Study the drawing (mm; zero at the part's minimum x, y, z) and answer. A direction names the side the tool comes from. Give positions to 0.01 mm unless a question says otherwise; leave off trailing zeros. Write each loop counter-clockwise with the first axis right and the second up, starting at its lowest first coordinate (ties: lowest second). Pieces come first, ordered by that corner, then holes. Notation, with made-up numbers: (-22, 33) - (-13, 33) arc R26 cw to (-13, 62) - close; hole circle Ø11 at (-1.5, -30). An arc over 180 degrees is marked (long way). Return JSON: item names as keys, results as strings.
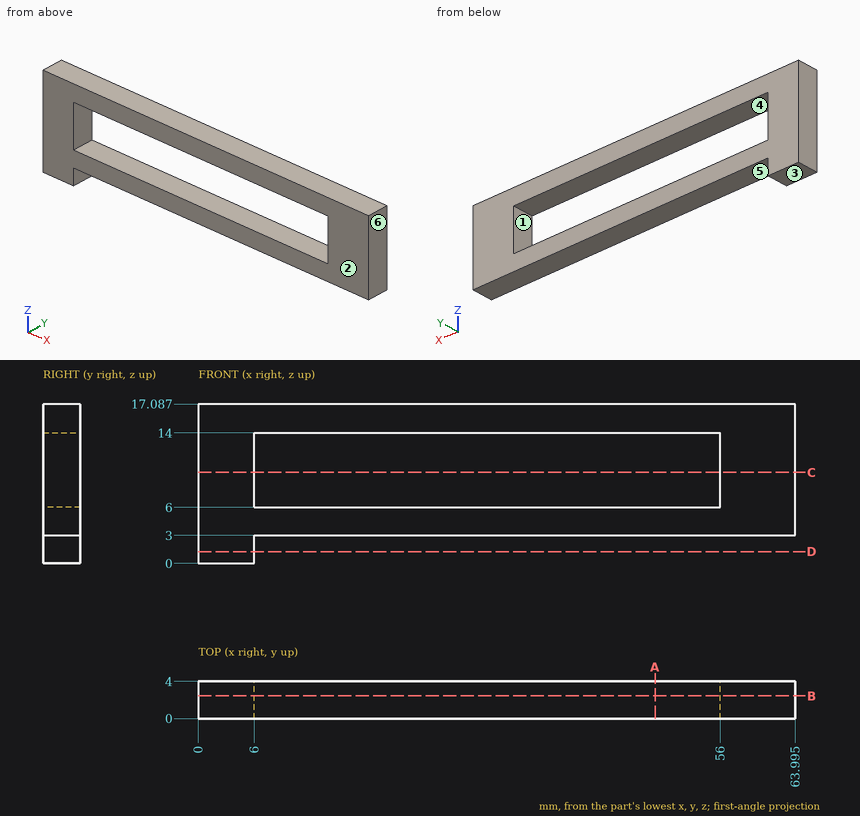
Item 1: The mould has two halves that part along Z. Classify the marked faces 1, 2 and 3: +Z half, -Z half, draft (parallel to the pull), parting line (faces both ways), or undercut.
Answer below:
{"face 1": "undercut", "face 2": "draft", "face 3": "-Z half"}
Item 2: A cutting plane is placed at A-A on x = 49. Determine the outline of the cut face in (y, z).
Answer below:
{"outline": "(0, 3) - (4, 3) - (4, 6) - (0, 6) - close; (0, 14) - (4, 14) - (4, 17.09) - (0, 17.09) - close"}
Item 3: A cutting plane is placed at B-B on y = 2.45. Determine the outline of the cut face in (x, z) (1 decimal).
Answer below:
{"outline": "(0, 0) - (6, 0) - (6, 3) - (64, 3) - (64, 17.1) - (0, 17.1) - close; hole (6, 6) - (56, 6) - (56, 14) - (6, 14) - close"}
Item 4: Consider L1, parallel to Z at x = 54, y = 0.75; L2, parallel to X at y = 0.7, z = 11.25 (1 decimal); L3, parallel to X at y = 0.2, z = 1.75. Determine where each line is inside the solid, lowest interval first.
Answer below:
{"L1": "z = 3 to 6, 14 to 17.09", "L2": "x = 0 to 6, 56 to 64", "L3": "x = 0 to 6"}
Item 5: For the marked faces 4, 5 and 6, determine the directions among +Z, -Z, +X, -X, +Y, -Y from which every point of the face is accessible in a straight line to the end or side of a thin tool.
Answer below:
{"face 4": "+Y, -Y", "face 5": "-Z, +X, +Y, -Y", "face 6": "+Z, -Z, +X, +Y, -Y"}
Item 6: A cutting plane is placed at C-C on z = 9.75. Determine the outline of the cut face in (x, y) (1 decimal).
Answer below:
{"outline": "(0, 0) - (6, 0) - (6, 4) - (0, 4) - close; (56, 0) - (64, 0) - (64, 4) - (56, 4) - close"}
Item 7: Flat-ended cylindrical pins translate along their axes: P1, Ø1.5, axis at y = 2, z = 1, coming from the +X side; P2, Ø1, axis at x = 13, z = 13, coming from the -Y side; P3, Ø1.2, axis at x = 45, y = 1, coming from the -Z side. Find the tip coordinate at first contact, or state that the pin passes through.
Answer below:
{"P1": "stops at x = 6", "P2": "passes through", "P3": "stops at z = 3"}
Item 8: A cutting plane is placed at D-D on z = 1.25. Determine the outline of the cut face in (x, y), then the cut area to 3 significant figures.
Answer below:
{"outline": "(0, 0) - (6, 0) - (6, 4) - (0, 4) - close", "area": "24.0 mm²"}
